Work out the finished part from the listing and answer in its coordinate system (mm). Face numbers are marked on the shaded views. Round coordinates to 2 decimals unless told otherwise and drop trailing zeros. Loops run counter-clockwise (first coordinate to the right, second up) from the corner with the lowest first, then second, coordinate; pieces in that order, holes last. Notation, with made-up numbers: (24.25, -1) - (38.25, -1) arc R10 ccw to (38.25, 10) - close; hole circle Ø11 at (-19, 89.25). An arc over 180 degrees is marked (long way). Return JSON: item names as keys, results as strings.
from build123d import *

# Parameters (mm, degrees)
BOX139_W               = 12
BOX139_H               = 16
BOX139_DEPTH           = 23
BOX139_PLACEMENT_ANGLE = 45
BOX141_W               = 6
BOX141_H               = 1
BOX141_DEPTH           = 1
BOX140_W               = 1
BOX140_H               = 1
BOX140_DEPTH           = 5
BOX140_PLACEMENT_ANGLE = 45
BOX136_W               = 12
BOX136_H               = 16
BOX136_DEPTH           = 23
BOX136_PLACEMENT_ANGLE = 45
BOX137_W               = 6
BOX137_H               = 1
BOX137_DEPTH           = 1
BOX138_W               = 1
BOX138_H               = 1
BOX138_DEPTH           = 5
BOX138_PLACEMENT_ANGLE = 45
BOX130_W               = 5
BOX130_H               = 16
BOX130_DEPTH           = 5
BOX130_PLACEMENT_ANGLE = 45
BOX131_W               = 5
BOX131_H               = 16
BOX131_DEPTH           = 5
BOX131_PLACEMENT_ANGLE = 45
BOX129_W               = 5
BOX129_H               = 16
BOX129_DEPTH           = 5
BOX129_PLACEMENT_ANGLE = 45
BOX034_W               = 45
BOX034_H               = 1
BOX034_DEPTH           = 19
BOX034_PLACEMENT_ANGLE = 45
BOX035_W               = 45
BOX035_H               = 1
BOX035_DEPTH           = 18
BOX035_PLACEMENT_ANGLE = 45
BOX142_W               = 12
BOX142_H               = 16
BOX142_DEPTH           = 23
BOX142_PLACEMENT_ANGLE = 45
BOX144_W               = 6
BOX144_H               = 1
BOX144_DEPTH           = 1
BOX143_W               = 1
BOX143_H               = 1
BOX143_DEPTH           = 5
BOX143_PLACEMENT_ANGLE = 45


with BuildPart() as box139:
    # Box139 → Box139 (new body)
    with BuildSketch(Plane.XY):
        with Locations((6, 8)):
            Rectangle(BOX139_W, BOX139_H)
    extrude(amount=BOX139_DEPTH)


with BuildPart() as box139_1:
    # Box139 placement: moved
    add(box139.part.moved(Location((22, -11.36, 22.5))).rotate(Axis((22, -11.36, 22.5), (-1, 0, 0)), BOX139_PLACEMENT_ANGLE))


with BuildPart() as cut052:
    # Box141 → Box141 (new body)
    with BuildSketch(Plane(origin=(23, 11, 22.2), x_dir=(1, 0, 0), z_dir=(0, 0, 1))):
        with Locations((3, 0.5)):
            Rectangle(BOX141_W, BOX141_H)
    extrude(amount=BOX141_DEPTH)

    # Cut052: cut Box139
    add(box139_1.part, mode=Mode.SUBTRACT)


with BuildPart() as cut052_1:
    # Cut052 placement: moved
    add(cut052.part.moved(Location((-12, -6.5, -5.7))))


with BuildPart() as fusion068:
    # Box140 → Box140 (new body)
    with BuildSketch(Plane.XY):
        with Locations((0.5, 0.5)):
            Rectangle(BOX140_W, BOX140_H)
    extrude(amount=BOX140_DEPTH)


with BuildPart() as fusion068_1:
    # Box140 placement: moved
    add(fusion068.part.moved(Location((13.5, 2, 14))).rotate(Axis((13.5, 2, 14), (-1, 0, 0)), BOX140_PLACEMENT_ANGLE))

    # Fusion068: union Cut052
    add(cut052_1.part)


with BuildPart() as fusion068_2:
    # Fusion068 placement: moved
    add(fusion068_1.part.moved(Location((12, 0, 0))))


with BuildPart() as box136:
    # Box136 → Box136 (new body)
    with BuildSketch(Plane.XY):
        with Locations((6, 8)):
            Rectangle(BOX136_W, BOX136_H)
    extrude(amount=BOX136_DEPTH)


with BuildPart() as box136_1:
    # Box136 placement: moved
    add(box136.part.moved(Location((22, -11.36, 22.5))).rotate(Axis((22, -11.36, 22.5), (-1, 0, 0)), BOX136_PLACEMENT_ANGLE))


with BuildPart() as cut051:
    # Box137 → Box137 (new body)
    with BuildSketch(Plane(origin=(23, 11, 22.2), x_dir=(1, 0, 0), z_dir=(0, 0, 1))):
        with Locations((3, 0.5)):
            Rectangle(BOX137_W, BOX137_H)
    extrude(amount=BOX137_DEPTH)

    # Cut051: cut Box136
    add(box136_1.part, mode=Mode.SUBTRACT)


with BuildPart() as cut051_1:
    # Cut051 placement: moved
    add(cut051.part.moved(Location((-12, -6.5, -5.7))))


with BuildPart() as fusion067:
    # Box138 → Box138 (new body)
    with BuildSketch(Plane.XY):
        with Locations((0.5, 0.5)):
            Rectangle(BOX138_W, BOX138_H)
    extrude(amount=BOX138_DEPTH)


with BuildPart() as fusion067_1:
    # Box138 placement: moved
    add(fusion067.part.moved(Location((13.5, 2, 14))).rotate(Axis((13.5, 2, 14), (-1, 0, 0)), BOX138_PLACEMENT_ANGLE))

    # Fusion067: union Cut051
    add(cut051_1.part)


with BuildPart() as box130:
    # Box130 → Box130 (new body)
    with BuildSketch(Plane.XY):
        with Locations((2.5, 8)):
            Rectangle(BOX130_W, BOX130_H)
    extrude(amount=BOX130_DEPTH)


with BuildPart() as box130_1:
    # Box130 placement: moved
    add(box130.part.moved(Location((35.5, -6.36, 22.5))).rotate(Axis((35.5, -6.36, 22.5), (-1, 0, 0)), BOX130_PLACEMENT_ANGLE))


with BuildPart() as box131:
    # Box131 → Box131 (new body)
    with BuildSketch(Plane.XY):
        with Locations((2.5, 8)):
            Rectangle(BOX131_W, BOX131_H)
    extrude(amount=BOX131_DEPTH)


with BuildPart() as box131_1:
    # Box131 placement: moved
    add(box131.part.moved(Location((11.5, -6.36, 22.5))).rotate(Axis((11.5, -6.36, 22.5), (-1, 0, 0)), BOX131_PLACEMENT_ANGLE))


with BuildPart() as box129:
    # Box129 → Box129 (new body)
    with BuildSketch(Plane.XY):
        with Locations((2.5, 8)):
            Rectangle(BOX129_W, BOX129_H)
    extrude(amount=BOX129_DEPTH)


with BuildPart() as box129_1:
    # Box129 placement: moved
    add(box129.part.moved(Location((23.5, -6.36, 22.5))).rotate(Axis((23.5, -6.36, 22.5), (-1, 0, 0)), BOX129_PLACEMENT_ANGLE))


with BuildPart() as box034:
    # Box034 → Box034 (new body)
    with BuildSketch(Plane.XY):
        with Locations((22.5, 0.5)):
            Rectangle(BOX034_W, BOX034_H)
    extrude(amount=BOX034_DEPTH)


with BuildPart() as box034_1:
    # Box034 placement: moved
    add(box034.part.moved(Location((0, -1, 11))).rotate(Axis((0, -1, 11), (-1, 0, 0)), BOX034_PLACEMENT_ANGLE))


with BuildPart() as cut048:
    # Box035 → Box035 (new body)
    with BuildSketch(Plane.XY):
        with Locations((22.5, 0.5)):
            Rectangle(BOX035_W, BOX035_H)
    extrude(amount=BOX035_DEPTH)


with BuildPart() as cut048_1:
    # Box035 placement: moved
    add(cut048.part.moved(Location((0, 25, 11))).rotate(Axis((0, 25, 11), (1, 0, 0)), BOX035_PLACEMENT_ANGLE))

    # Fusion059: union Box034
    add(box034_1.part)

    # Cut046: cut Box129
    add(box129_1.part, mode=Mode.SUBTRACT)

    # Cut047: cut Box131
    add(box131_1.part, mode=Mode.SUBTRACT)

    # Cut048: cut Box130
    add(box130_1.part, mode=Mode.SUBTRACT)


with BuildPart() as box142:
    # Box142 → Box142 (new body)
    with BuildSketch(Plane.XY):
        with Locations((6, 8)):
            Rectangle(BOX142_W, BOX142_H)
    extrude(amount=BOX142_DEPTH)


with BuildPart() as box142_1:
    # Box142 placement: moved
    add(box142.part.moved(Location((22, -11.36, 22.5))).rotate(Axis((22, -11.36, 22.5), (-1, 0, 0)), BOX142_PLACEMENT_ANGLE))


with BuildPart() as cut053:
    # Box144 → Box144 (new body)
    with BuildSketch(Plane(origin=(23, 11, 22.2), x_dir=(1, 0, 0), z_dir=(0, 0, 1))):
        with Locations((3, 0.5)):
            Rectangle(BOX144_W, BOX144_H)
    extrude(amount=BOX144_DEPTH)

    # Cut053: cut Box142
    add(box142_1.part, mode=Mode.SUBTRACT)


with BuildPart() as cut053_1:
    # Cut053 placement: moved
    add(cut053.part.moved(Location((-12, -6.5, -5.7))))


with BuildPart() as fusion070:
    # Box143 → Box143 (new body)
    with BuildSketch(Plane.XY):
        with Locations((0.5, 0.5)):
            Rectangle(BOX143_W, BOX143_H)
    extrude(amount=BOX143_DEPTH)


with BuildPart() as fusion070_1:
    # Box143 placement: moved
    add(fusion070.part.moved(Location((13.5, 2, 14))).rotate(Axis((13.5, 2, 14), (-1, 0, 0)), BOX143_PLACEMENT_ANGLE))

    # Fusion069: union Cut053
    add(cut053_1.part)


with BuildPart() as fusion070_2:
    # Fusion069 placement: moved
    add(fusion070_1.part.moved(Location((24, 0, 0))))

    # Fusion070: union Fusion068, Fusion067, Cut048
    add(fusion068_2.part)
    add(fusion067_1.part)
    add(cut048_1.part)


solid = fusion070_2.part
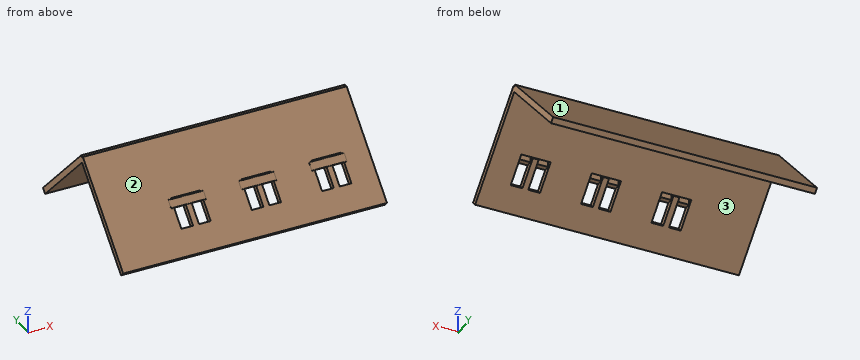
1) Section A-A (y = 4) is taken. Give the vertices of the cut face in (x, z).
Verdict:
{"outline": "(0, 14.59) - (11.5, 14.59) - (11.5, 16) - (0, 16) - close; (13.5, 14.59) - (14.5, 14.59) - (14.5, 16) - (13.5, 16) - close; (16.5, 14.59) - (23.5, 14.59) - (23.5, 16) - (16.5, 16) - close; (25.5, 14.59) - (26.5, 14.59) - (26.5, 16) - (25.5, 16) - close; (28.5, 14.59) - (35.5, 14.59) - (35.5, 16) - (28.5, 16) - close; (37.5, 14.59) - (38.5, 14.59) - (38.5, 16) - (37.5, 16) - close; (40.5, 14.59) - (45, 14.59) - (45, 16) - (40.5, 16) - close"}
2) Determine the mould class of the marked faces 1, 2 and 3 for opening direction Y: pulls with the +Y half, pulls with the -Y half, needs draft (parallel to the pull), parting line crosses it, or undercut.
Verdict:
{"face 1": "pulls with the +Y half", "face 2": "pulls with the -Y half", "face 3": "undercut"}
3) Flat-ended cylindrical pins translate along their axes: pin 1 (5 mm diameter, centred on x = 7.5, z = 16, fed in from -Y); pin 2 (0.5 mm diameter, centred on x = 36.5, z = 17, fed in from +Y); pin 3 (5 mm diameter, centred on x = 23, y = 7, fed in from +Z). Find the tip coordinate at first contact, or state that the pin passes through.
Verdict:
{"pin 1": "stops at y = 1.5", "pin 2": "stops at y = 20.66", "pin 3": "stops at z = 21.5"}
4) Find the intervals of material crossed by L1, parallel to Y at x = 5, z = 15.5; L2, parallel to Y at x = 6.5, z = 15; L3, parallel to Z at x = 42, y = 12.5, in increasing order.
Verdict:
{"L1": "y = 3.5 to 4.91, 20.5 to 21.91", "L2": "y = 3 to 4.41, 21 to 22.41", "L3": "z = 23.09 to 24.37"}
5) Section C-C (z = 18.5) is taken. Give the vertices of the cut face in (x, y).
Verdict:
{"outline": "(0, 6.5) - (45, 6.5) - (45, 7.91) - (0, 7.91) - close; (0, 17.5) - (45, 17.5) - (45, 18.91) - (0, 18.91) - close"}
6) Section B-B (x = 24) is taken. Count the separate pieces of the cut face and the enclosed holes in it, and give its area (3 significant figures).
Verdict:
{"separate pieces": "3", "enclosed holes": "0", "area": "32.2 mm2"}
